The listing builds one solid part. Answer for the finished solid, in the listing's coordinates (mm). A direction names the side the tool comes from. Give positions to 0.01 mm unless a question says otherwise; leave off trailing zeros. Order: outer loops, then holes, each group sorted by start corner. A loop starts at its lowest first (then second) coordinate and runs counter-clockwise, first axis right, second up. Notation, with made-up numbers: (55.5, 85) -> (81.5, 85) arc R16 ccw to (81.5, 107) -> close; hole circle Ø1 at (54.5, 38). An arc over 180 degrees is marked (long way). One line per question, with ' | ' between items. Start each with the question number.
```python
from build123d import *

# Parameters (mm, degrees)
BOSS_EXTRUDE1_DEPTH      = 1
BOSS_EXTRUDE2_DEPTH      = 11
BOSS_EXTRUDE3_DEPTH      = 5
BOSS_EXTRUDE3_DEPTH_BACK = 3
SKETCH3_W                = 50
SKETCH3_H                = 7
CUT_EXTRUDE3_DEPTH       = 25
SKETCH5_W                = 50
SKETCH5_H                = 7
CUT_EXTRUDE4_DEPTH       = 25
SKETCH6_W                = 50
SKETCH6_H                = 7
CUT_EXTRUDE5_DEPTH       = 25
SKETCH8_R                = 1.5
BOSS_EXTRUDE5_DEPTH      = 1
BOSS_EXTRUDE10_DEPTH     = 3


with BuildPart() as part:
    # Sketch1 → Boss-Extrude1 (new body)
    with BuildSketch(Plane(origin=(0, 0, 0), x_dir=(1, 0, 0), z_dir=(0, 1, 0))):
        Polygon((243.304219773, -116.484791866), (254.809280576, -136.408896139), (442.602090749, -136.409305398), (444.621046679, -132.925433223), (441.749040748, -132.925433223), (449.516726723, -119.471406457), (450.964695297, -121.978953122), (452.699916621, -118.984688017), (358.778179035, 43.666038066), (335.767496284, 43.666038066), align=None)
        Polygon((428.113670919, -116.417164681), (266.439108268, -116.428009241), (347.273609729, 23.609230825), align=None, mode=Mode.SUBTRACT)
    extrude(amount=BOSS_EXTRUDE1_DEPTH)

    # Sketch1_9 → Boss-Extrude2 (add)
    # profile 1 of 2: a face of its own
    with BuildSketch(Plane(origin=(0, 0, 0), x_dir=(1, 0, 0), z_dir=(0, 1, 0))):
        Polygon((229.159432547, -134.984249184), (231.716666588, -139.412373829), (462.829865412, -139.412373829), (465.38624875, -134.984588004), (349.829542096, 65.165499075), (344.716133219, 65.165499075), align=None)
        Polygon((251.922647988, -136.4093054), (233.446303399, -136.408896139), (232.623553959, -134.984217358), (241.860901688, -118.984688019), align=None, mode=Mode.SUBTRACT)
        Polygon((442.602090749, -136.409305398), (254.809280576, -136.408896139), (243.304219773, -116.484791866), (335.767496284, 43.666038066), (358.778179035, 43.666038066), (461.938967957, -134.984588004), (461.116393748, -136.409305398), align=None, mode=Mode.SUBTRACT)
        Polygon((348.096628302, 62.164013367), (357.334800991, 46.166038067), (337.210874326, 46.166038067), (346.44844193, 62.165948237), align=None, mode=Mode.SUBTRACT)
    # profile 2 of 2: a face of its own
    with BuildSketch(Plane(origin=(0, 0, 0), x_dir=(1, 0, 0), z_dir=(0, 1, 0))):
        Polygon((441.749040748, -132.925433223), (444.621046679, -132.925433223), (450.964695297, -121.978953122), (449.516726723, -119.471406457), align=None)
    extrude(amount=BOSS_EXTRUDE2_DEPTH)

    # Sketch1_10 → Boss-Extrude3 (add, two sides: drawn at the far end of the back side and taken through both)
    with BuildSketch(Plane(origin=(0, 0, 0), x_dir=(1, 0, 0), z_dir=(0, 1, 0)).offset(-BOSS_EXTRUDE3_DEPTH_BACK)):
        Polygon((229.159432547, -134.984249184), (231.716666588, -139.412373829), (462.829865412, -139.412373829), (465.38624875, -134.984588004), (349.829542096, 65.165499075), (344.716133219, 65.165499075), align=None)
        Polygon((251.922647988, -136.4093054), (233.446303399, -136.408896139), (232.623553959, -134.984217358), (241.860901688, -118.984688019), align=None, mode=Mode.SUBTRACT)
        Polygon((442.602090749, -136.409305398), (254.809280576, -136.408896139), (243.304219773, -116.484791866), (335.767496284, 43.666038066), (358.778179035, 43.666038066), (452.699916621, -118.984688017), (461.938967957, -134.984588004), (461.116393748, -136.409305398), align=None, mode=Mode.SUBTRACT)
        Polygon((348.096628302, 62.164013367), (357.334800991, 46.166038067), (337.210874326, 46.166038067), (346.44844193, 62.165948237), align=None, mode=Mode.SUBTRACT)
    extrude(amount=BOSS_EXTRUDE3_DEPTH + BOSS_EXTRUDE3_DEPTH_BACK)

    # Sketch3 → Cut-Extrude3 (cut)
    with BuildSketch(Plane(origin=(290.589645397, 0, -167.772009994), x_dir=(-0.49999999999998745, 0, -0.8660254037844459), z_dir=(0.8660254037844459, 0, -0.49999999999998745))):
        with Locations((-236.592990632, -3)):
            Rectangle(SKETCH3_W, SKETCH3_H)
    extrude(amount=-CUT_EXTRUDE3_DEPTH, mode=Mode.SUBTRACT)

    # Sketch5 → Cut-Extrude4 (cut)
    with BuildSketch(Plane.XY.offset(139.412373829)):
        with Locations((347.273266, -3)):
            Rectangle(SKETCH5_W, SKETCH5_H)
    extrude(amount=-CUT_EXTRUDE4_DEPTH, mode=Mode.SUBTRACT)

    # Sketch6 → Cut-Extrude5 (cut)
    with BuildSketch(Plane(origin=(230.319375797, 0, 132.975171838), x_dir=(-0.5000006154012504, 0, 0.8660250484820695), z_dir=(-0.8660250484820695, 0, -0.5000006154012504))):
        with Locations((-113.2366748, -3)):
            Rectangle(SKETCH6_W, SKETCH6_H)
    extrude(amount=-CUT_EXTRUDE5_DEPTH, mode=Mode.SUBTRACT)

    # Sketch8 → Boss-Extrude5 (add)
    with BuildSketch(Plane.XZ.offset(3)):
        Polygon((349.829542096, -65.165499075), (465.38624875, 134.984588004), (462.829865412, 139.412373829), (231.716666588, 139.412373829), (229.159432547, 134.984249184), (344.716133219, -65.165499075), align=None)
        with Locations(Location((395.323540807, 98.692824234, 0), (0, 0, 270))):
            Circle(SKETCH8_R, mode=Mode.SUBTRACT)
        with Locations(Location((348.301285092, 15.863526629, 0), (0, 0, 270))):
            Circle(SKETCH8_R, mode=Mode.SUBTRACT)
        with Locations(Location((299.654911442, 97.241681781, 0), (0, 0, 270))):
            Circle(SKETCH8_R, mode=Mode.SUBTRACT)
        Polygon((450.14703547, 123.280701064), (452.699916621, 118.984688017), (461.938967957, 134.984588004), (461.116393748, 136.409305398), (442.602090749, 136.409305398), (445.226665069, 131.986443715), (401.697951811, 107.384591709), (406.618322212, 98.678849058), align=None, mode=Mode.SUBTRACT)
        Polygon((322.273266, 116.424264082), (294.358218631, 68.061097964), (319.354499366, 24.757680453), (376.473657317, 26.969372805), (401.47267951, 70.271207531), (372.273266, 116.420910258), align=None, mode=Mode.SUBTRACT)
        Polygon((233.446303399, 136.408896139), (251.922647988, 136.4093054), (241.860901688, 118.984688019), (232.623553959, 134.984217358), align=None, mode=Mode.SUBTRACT)
        Polygon((337.210874326, -46.166038067), (357.334800991, -46.166038067), (348.096628302, -62.164013367), (346.44844193, -62.165948237), align=None, mode=Mode.SUBTRACT)
    extrude(amount=BOSS_EXTRUDE5_DEPTH)

    # Sketch12 → Boss-Extrude10 (add)
    with BuildSketch(Plane(origin=(0, -3, 0), x_dir=(1, 0, 0), z_dir=(0, 1, 0))):
        with BuildLine():
            Line((347.417900212, -11.962292061), (347.307477102, -11.47463774))
            ThreePointArc((347.307477102, -11.47463774), (345.119304576, -12.681546113), (343.912396203, -14.869718639))
            Line((343.912396203, -14.869718639), (344.400050524, -14.980141749))
            ThreePointArc((344.400050524, -14.980141749), (345.472857967, -13.035099504), (347.417900212, -11.962292061))
        make_face()
        with BuildLine():
            ThreePointArc((352.69017398, -14.869718639), (351.483265607, -12.681546113), (349.295093082, -11.47463774))
            Line((349.295093082, -11.47463774), (349.184669972, -11.962292061))
            ThreePointArc((349.184669972, -11.962292061), (351.129712216, -13.035099504), (352.202519659, -14.980141749))
            Line((352.202519659, -14.980141749), (352.69017398, -14.869718639))
        make_face()
        with BuildLine():
            ThreePointArc((349.295093082, -20.252415518), (351.483265607, -19.045507144), (352.69017398, -16.857334619))
            Line((352.69017398, -16.857334619), (352.202519659, -16.746911509))
            ThreePointArc((352.202519659, -16.746911509), (351.129712216, -18.691953754), (349.184669972, -19.764761197))
            Line((349.184669972, -19.764761197), (349.295093082, -20.252415518))
        make_face()
        with BuildLine():
            Line((344.400050524, -16.746911509), (343.912396203, -16.857334619))
            ThreePointArc((343.912396203, -16.857334619), (345.119304576, -19.045507144), (347.307477102, -20.252415518))
            Line((347.307477102, -20.252415518), (347.417900212, -19.764761197))
            ThreePointArc((347.417900212, -19.764761197), (345.472857967, -18.691953754), (344.400050524, -16.746911509))
        make_face()
        with BuildLine():
            Line((394.440155927, -94.791589666), (394.329732817, -94.303935345))
            ThreePointArc((394.329732817, -94.303935345), (392.141560292, -95.510843719), (390.934651919, -97.699016244))
            Line((390.934651919, -97.699016244), (391.4247896, -97.798542945))
            ThreePointArc((391.4247896, -97.798542945), (392.499067689, -95.860448622), (394.440155927, -94.791589666))
        make_face()
        with BuildLine():
            ThreePointArc((399.712429696, -97.699016244), (398.505521323, -95.510843719), (396.317348797, -94.303935345))
            Line((396.317348797, -94.303935345), (396.206925687, -94.791589666))
            ThreePointArc((396.206925687, -94.791589666), (398.151967932, -95.864397109), (399.224775375, -97.809439354))
            Line((399.224775375, -97.809439354), (399.712429696, -97.699016244))
        make_face()
        with BuildLine():
            ThreePointArc((396.317348797, -103.081713123), (398.505521323, -101.874804749), (399.712429696, -99.686632224))
            Line((399.712429696, -99.686632224), (399.224775375, -99.576209114))
            ThreePointArc((399.224775375, -99.576209114), (398.151967932, -101.521251359), (396.206925687, -102.594058802))
            Line((396.206925687, -102.594058802), (396.317348797, -103.081713123))
        make_face()
        with BuildLine():
            Line((391.422306239, -99.576209114), (390.934651919, -99.686632224))
            ThreePointArc((390.934651919, -99.686632224), (392.141560292, -101.874804749), (394.329732817, -103.081713123))
            Line((394.329732817, -103.081713123), (394.440155927, -102.594058802))
            ThreePointArc((394.440155927, -102.594058802), (392.495113683, -101.521251359), (391.422306239, -99.576209114))
        make_face()
        with BuildLine():
            ThreePointArc((298.661103452, -92.852792892), (296.472930927, -94.059701266), (295.266022553, -96.247873791))
            Line((295.266022553, -96.247873791), (295.753676874, -96.358296901))
            ThreePointArc((295.753676874, -96.358296901), (296.826484317, -94.413254657), (298.771526562, -93.340447213))
            Line((298.771526562, -93.340447213), (298.661103452, -92.852792892))
        make_face()
        with BuildLine():
            ThreePointArc((304.043800331, -96.247873791), (302.836891957, -94.059701266), (300.648719432, -92.852792892))
            Line((300.648719432, -92.852792892), (300.538296322, -93.340447213))
            ThreePointArc((300.538296322, -93.340447213), (302.483338567, -94.413254657), (303.55614601, -96.358296901))
            Line((303.55614601, -96.358296901), (304.043800331, -96.247873791))
        make_face()
        with BuildLine():
            Line((300.538296322, -101.142916349), (300.648719432, -101.63057067))
            ThreePointArc((300.648719432, -101.63057067), (302.836891957, -100.423662297), (304.043800331, -98.235489771))
            Line((304.043800331, -98.235489771), (303.55614601, -98.125066661))
            ThreePointArc((303.55614601, -98.125066661), (302.483338567, -100.070108906), (300.538296322, -101.142916349))
        make_face()
        with BuildLine():
            Line((295.753676874, -98.125066661), (295.266022553, -98.235489771))
            ThreePointArc((295.266022553, -98.235489771), (296.472930927, -100.423662297), (298.661103452, -101.63057067))
            Line((298.661103452, -101.63057067), (298.771526562, -101.142916349))
            ThreePointArc((298.771526562, -101.142916349), (296.826484317, -100.070108906), (295.753676874, -98.125066661))
        make_face()
    extrude(amount=BOSS_EXTRUDE10_DEPTH)


solid = part.part
```
(1) The part is cut by section D-D on z = 42. Determine the outline of the cut face in (x, y), plus the area to 3 significant figures.
(2) Determine the mould class of faces 1 (the face through (306.29, 0.72, 47.39)), 2 (the face through (273, 0, 97)), 3 (the face through (447, 11, 127)) for opening direction Y: pulls with the +Y half, pulls with the -Y half, needs draft (parallel to the pull), parting line crosses it, or undercut.
(3) The part is cut by section C-C on z = 89.5. Determine the outline of the cut face in (x, y).
(4) The part is cut by section A-A on y = 5.75. Determine the outline of the cut face in (x, z), plus the area to 3 significant figures.
(5) The part is cut by section B-B on x = 409.5. Determine the outline of the cut face in (y, z), plus the area to 3 significant figures.
(6) For faces 4 (the face through (390.9, 0.17, 18.64)), 5 (the face through (445.69, 5.93, 126.1)), 6 (the face through (399, 0.5, 43)), determine the directions among +Z, -Z, +X, -X, +Y, -Y from which every point of the face is accessible in a straight line to the end or side of a thin tool.
(7) Consider line 1 (Y direction, x = 266, z = 115); line 2 (X direction, y = 10.25, z = -9.5); line 3 (Z direction, x = 369.5, y = 8.5). Determine where each line is inside the solid, lowest interval first.
(8) Given P1, Ø3, axis at x = 393, z = 101.5, coming from the +Y side; P2, Ø2, axis at x = 273.5, z = 93, coming from the +Y side; P3, Ø5, axis at x = 333, z = 29, coming from the +Y side; P4, Ø5, axis at x = 299.65, z = 97.24, coming from the +Y side, each flat-ended and moving along its own axis, determine where each tip first touches the part or whether it passes through.
Result sheet:
1) outline: (282.84, -4) -> (309.4, -4) -> (309.4, -3) -> (282.84, -3) -> close; (282.84, 0.5) -> (309.4, 0.5) -> (309.4, 1) -> (286.31, 1) -> (286.31, 11) -> (282.84, 11) -> close; (385.15, -4) -> (411.7, -4) -> (411.7, -3) -> (385.15, -3) -> close; (385.15, 0.5) -> (411.7, 0.5) -> (411.7, 11) -> (408.25, 11) -> (408.25, 1) -> (385.15, 1) -> close | area: 149 mm^2
2) face 1: needs draft | face 2: undercut | face 3: pulls with the +Y half
3) outline: (255.42, -4) -> (306.73, -4) -> (306.73, -3) -> (258.88, -3) -> (258.88, 0) -> (281.98, 0) -> (281.98, 1) -> (258.88, 1) -> (258.88, 11) -> (255.42, 11) -> close; (389.31, -4) -> (439.13, -4) -> (439.13, 11) -> (435.67, 11) -> (435.67, 1) -> (412.57, 1) -> (412.57, 0) -> (435.67, 0) -> (435.67, -3) -> (389.31, -3) -> close
4) outline: (229.16, 134.98) -> (344.72, -65.17) -> (349.83, -65.17) -> (465.39, 134.98) -> (462.83, 139.41) -> (231.72, 139.41) -> close; (441.75, 132.93) -> (449.52, 119.47) -> (450.96, 121.98) -> (444.62, 132.93) -> close; hole (232.62, 134.98) -> (241.86, 118.98) -> (251.92, 136.41) -> (233.45, 136.41) -> close; hole (243.3, 116.48) -> (335.77, -43.67) -> (358.78, -43.67) -> (461.94, 134.98) -> (461.12, 136.41) -> (442.6, 136.41) -> (254.81, 136.41) -> close; hole (337.21, -46.17) -> (346.45, -62.17) -> (348.1, -62.16) -> (357.33, -46.17) -> close | area: 2,240 mm^2
5) outline: (-4, 38.19) -> (-3, 38.19) -> (-3, 100.31) -> (-4, 100.31) -> close; (-4, 111.79) -> (-3, 111.79) -> (-3, 136.41) -> (0, 136.41) -> (0, 116.42) -> (1, 116.42) -> (1, 136.41) -> (11, 136.41) -> (11, 139.41) -> (-4, 139.41) -> close; (0, 65.64) -> (0.5, 65.64) -> (0.5, 38.19) -> (11, 38.19) -> (11, 44.17) -> (1, 44.17) -> (1, 84.18) -> (0, 84.18) -> close | area: 244 mm^2
6) face 4: +X | face 5: +Y | face 6: none
7) line 1: y = -4 to -3, 0 to 1 | line 2: x = 312.58 to 316.04, 378.51 to 381.97 | line 3: z = -31.1 to -25.1, 136.41 to 139.41
8) P1: stops at y = 0 | P2: stops at y = 1 | P3: passes through | P4: stops at y = -3
